Solid Edge part; units mm, degrees
sketch "Sketch1" plane through (0, 0, 0) normal (1, 0, 0) x (0, 1, 0)
  line L0 (41, 30) -> (-41, 30)
  line L1 (-41, 30) -> (-41, 10)
  line L2 (-41, 10) -> (-32, 10)
  line L3 (-32, 10) -> (-32, -20)
  line L4 (-32, -20) -> (-18, -20)
  line L5 (-18, -20) -> (-8.9199, -10.9199)
  arc A0 (-8.9199, -10.9199) -> (8.9199, -10.9199) centre (0, 0) cw
  line L6 (8.9199, -10.9199) -> (18, -20)
  line L7 (18, -20) -> (32, -20)
  line L8 (32, -20) -> (32, 10)
  line L9 (32, 10) -> (41, 10)
  line L10 (41, 10) -> (41, 30)
  dimension "D1" = 41
extrude "Protrusion1" add sketch "Sketch1" along normal mid plane 64
fillet "Round1" radius 12 2 edges at (0, -32, 10) (0, 32, 10)
CAD build for the part. Positions are in the model's coordinates, mm. A direction names the side the tool comes from. Coordinates: 2 decimals unless noted, no trailing zeros. Write each loop counter-clockwise with the first axis right and the second up, starting at its lowest first coordinate (ties: lowest second). Pieces come first, ordered by that corner, then holes. Notation, with made-up numbers: M 78.5,48.5 L 120.5,48.5 A13 ccw 120.5,64.5 Z; hole C 14.5,72.5 d4. An arc over 180 degrees is marked long. Answer as a JSON object with one key per item and string values. Group by question number.
1) Pin check, flat tips, straight feed: pin 1 Ø1 at (x, y) = (-3, 8.5) entering from -Z; pin 2 Ø4 at (x, z) = (21, -10.5) entering from +Y; pin 3 Ø10 at (x, z) = (6, 3.5) entering from +Y. Stop position of each tip, or through.
2) Wall check: line 1 (Y direction, x = -6, z = 0); line 2 (Y direction, x = 6, z = 7); line 3 (Z direction, x = 16.5, y = 0.5). Give the ranges that are in metal, low to high. Write a range as from..to.
3) Saw through at A-A (x = -23). Write the cut outline in (y, z).
4) Saw through at C-C (y = 0). Write the cut outline in (x, z).
5) Saw through at B-B (z = 0). Write the cut outline in (x, y), plus the area to 3 significant figures.
6) Mould opens along Y. For faces 1 (the face through (0, 13, -15)), 2 (the face through (0.448, 34.581, 5.817)), 3 (the face through (32, -1, 16)) say: +Y half, -Y half, draft (parallel to the pull), parting line (faces both ways), or undercut.
7) Tool access for faces 4 (the face through (0, 32, -11)), 5 (the face through (0, -14, -16)), 6 (the face through (0, -32, -11)): list every direction of +Z, -Z, +X, -X, +Y, -Y with a clear straight run to the whole face (end or side of a thin tool).
Values follow:
{
 "1": {"pin 1": "stops at z = -11", "pin 2": "stops at y = 32", "pin 3": "stops at y = 37.55"},
 "2": {"line 1": "y = -32.11..-14.1, 14.1..32.11", "line 2": "y = -35.65..-12.24, 12.24..35.65", "line 3": "z = 14.09..30"},
 "3": {"outline": "M -41,10 A12 cw -32,-1.62 L -32,-20 L -18,-20 L -8.92,-10.92 A14.1 cw long 8.92,-10.92 L 18,-20 L 32,-20 L 32,-1.62 A12 cw 41,10 L 41,30 L -41,30 Z"},
 "4": {"outline": "M -32,14.1 L 32,14.1 L 32,30 L -32,30 Z"},
 "5": {"outline": "M -32,-32.11 L 32,-32.11 L 32,-14.1 L -32,-14.1 Z; M -32,14.1 L 32,14.1 L 32,32.11 L -32,32.11 Z", "area": "2,310 mm2"},
 "6": {"face 1": "undercut", "face 2": "+Y half", "face 3": "draft"},
 "7": {"face 4": "-Z, +X, -X, +Y", "face 5": "-Z, +X, -X", "face 6": "-Z, +X, -X, -Y"}
}
